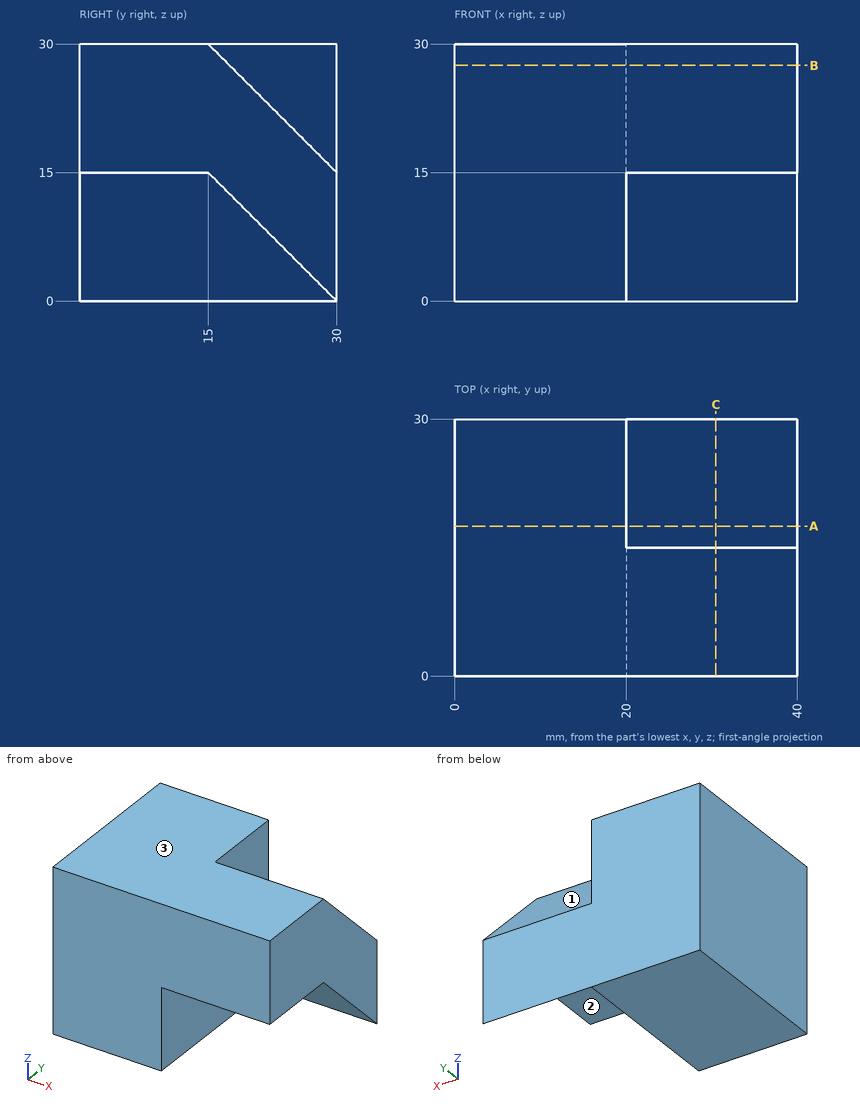
Design review of the part shown in the three views and the two pictorial views. Dimensions are in mm from the part's minimum x, y and z. A direction names the side the tool comes from. Coordinates: 2 decimals unless noted, no trailing zeros. Write each loop counter-clockwise with the first axis right and the second up, starting at its lowest first coordinate (ties: lowest second). Pieces come first, ordered by that corner, then holes.
1) We need section C-C on x = 30.5. State the section outline as (y, z) points, then the cut area to 3 significant figures.
2) We need section A-A on y = 17.5. State the section outline as (x, z) points.
3) We need section B-B on z = 27.5. State the section outline as (x, y) points, then the cut area to 3 significant figures.
4) Machinability: for the marked faces 1, 2 and 3, which of the approach directions +Z, -Z, +X, -X, +Y, -Y give a long, thin tool a straight path to every point of the face, cutting with its end or side? Answer none if there is none.
5) Clearance check with flat-ended pins moving along their axes: pin 1 Ø7.5 at (y, z) = (17.5, 10) entering from +X; pin 2 Ø2 at (x, y) = (27.5, 26.5) entering from -Z; pin 3 Ø2 at (x, z) = (26.5, 20.5) entering from +Y; pin 4 Ø7.5 at (x, y) = (34, 9) entering from -Z. State where each tip first meets the part, or that it passes through.
6) To check wall thickness, follow probe 1 along Z at (x, y) = (37, 13); probe 2 along X at (y, z) = (16.5, 4.25); probe 3 along Y at (x, z) = (38.5, 16). State the ranges of each line that lie inside material, in increasing order.
Answer list:
1. outline: (0, 15) - (15, 15) - (30, 0) - (30, 15) - (15, 30) - (0, 30) - close
1. area: 450 mm2
2. outline: (0, 0) - (20, 0) - (20, 12.5) - (40, 12.5) - (40, 27.5) - (20, 27.5) - (20, 30) - (0, 30) - close
3. outline: (0, 0) - (40, 0) - (40, 17.5) - (20, 17.5) - (20, 30) - (0, 30) - close
3. area: 950 mm2
4. face 1: +Z, +X, +Y
4. face 2: -Z, +X, -Y
4. face 3: +Z, +X, -X, +Y, -Y
5. pin 1: stops at x = 40
5. pin 2: stops at z = 2.5
5. pin 3: stops at y = 25.5
5. pin 4: stops at z = 15
6. probe 1: z = 15 to 30
6. probe 2: x = 0 to 20
6. probe 3: y = 0 to 29
